Drawing for the job (mm, zero at the part's lowest x, y, z). A direction names the side the tool comes from. Round coordinates to 2 decimals unless told otherwise and drop trailing zeros. Order: outer loops, then holes, each group sorted by start corner. A loop starts at its lowest first (then second) coordinate and runs counter-clockwise, first axis right, second up. Notation, with made-up numbers: M 69.5,71.5 L 95.5,71.5 A25 cw 95.5,91.5 Z; hole C -33.75,84.5 d5. An arc over 180 degrees is marked long. One line per item, written item: value. Start each with the question number.
Item 1: Pin check, flat tips, straight feed: pin 1 (5.5 mm diameter, centred on x = 10, z = 3, fed in from +Y); pin 2 (2.5 mm diameter, centred on y = 1, z = 9.5, fed in from +X); pin 3 (5.5 mm diameter, centred on x = 11, z = 12.5, fed in from +Y); pin 4 (2.5 mm diameter, centred on x = 11, z = 11, fed in from -Y). Stop position of each tip, or through.
Item 2: Two-plate mould, pull along X, no slides. Class the marked faces 4, 5 and 6: +X half, -X half, draft (parallel to the pull), parting line (faces both ways), or undercut.
Item 3: Band-saw the part on D-D, the plane z = 8.25. Write the cut outline in (x, y).
Item 4: Probe L1, parallel to Y at x = 15.5, z = 6.5; L2, parallel to Y at x = 9.25, z = 6; L3, parallel to X at y = 1.5, z = 16.25. List the from-to ranges inside material, lowest first.
Item 5: Band-saw the part on B-B, the plane y = 2. Write the cut outline in (x, z).
Item 6: Tool access for the marked faces 1, 2 and 3: list every direction of +Z, -Z, +X, -X, +Y, -Y with a clear straight run to the whole face (end or side of a thin tool).
Item 7: Band-saw the part on C-C, the plane z = 11. Write the cut outline in (x, y), then the cut area to 3 significant figures.
Item 8: Band-saw the part on A-A, the plane x = 11. Write the cut outline in (y, z), then the cut area to 3 significant figures.
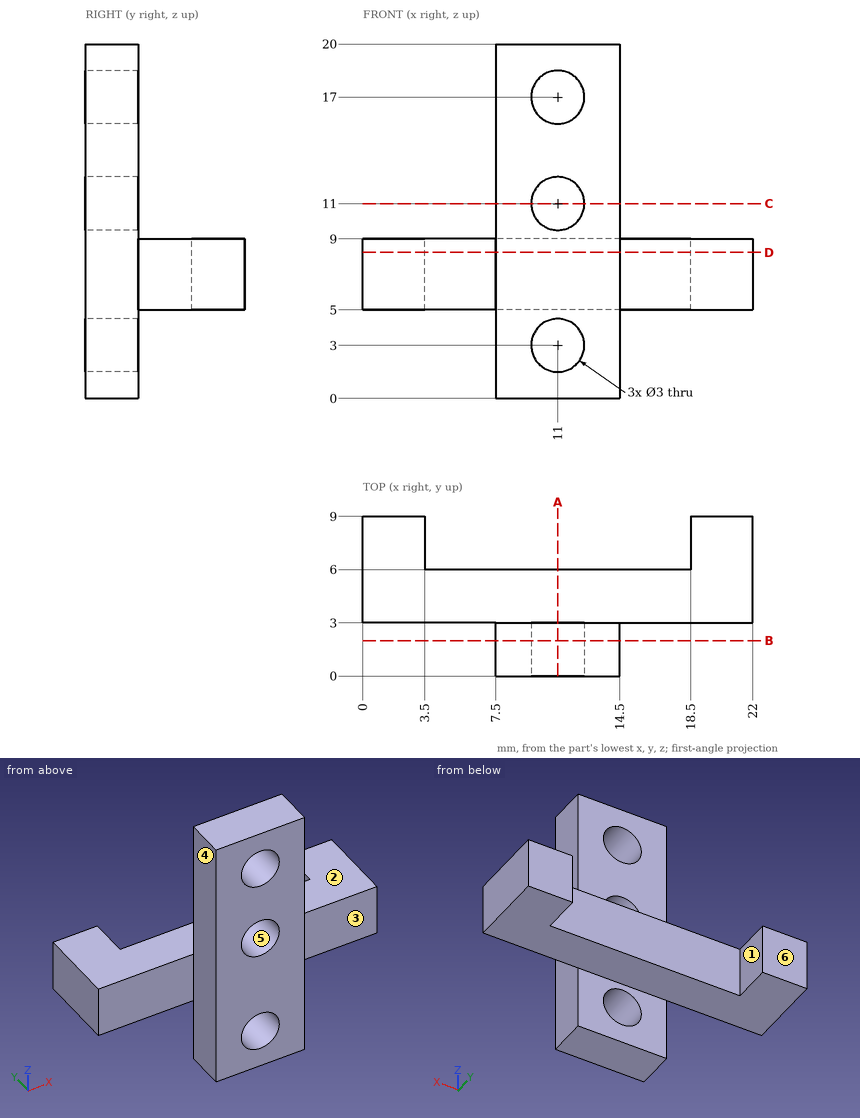
Output:
1. pin 1: stops at y = 6
1. pin 2: stops at x = 14.5
1. pin 3: stops at y = 3
1. pin 4: passes through
2. face 4: -X half
2. face 5: undercut
2. face 6: draft
3. outline: M 0,3 L 7.5,3 L 7.5,0 L 14.5,0 L 14.5,3 L 22,3 L 22,9 L 18.5,9 L 18.5,6 L 3.5,6 L 3.5,9 L 0,9 Z
4. L1: y = 3 to 6
4. L2: y = 0 to 6
4. L3: x = 7.5 to 9.7, 12.3 to 14.5
5. outline: M 7.5,0 L 14.5,0 L 14.5,20 L 7.5,20 Z; hole C 11,3 d3; hole C 11,11 d3; hole C 11,17 d3
6. face 1: +Z, -Z, +Y
6. face 2: +Z, +X, -X, +Y
6. face 3: +Z, -Z, +X, -Y
7. outline: M 7.5,0 L 9.5,0 L 9.5,3 L 7.5,3 Z; M 12.5,0 L 14.5,0 L 14.5,3 L 12.5,3 Z
7. area: 12.0 mm²
8. outline: M 0,0 L 3,0 L 3,1.5 L 0,1.5 Z; M 0,4.5 L 3,4.5 L 3,5 L 6,5 L 6,9 L 3,9 L 3,9.5 L 0,9.5 Z; M 0,12.5 L 3,12.5 L 3,15.5 L 0,15.5 Z; M 0,18.5 L 3,18.5 L 3,20 L 0,20 Z
8. area: 45.0 mm²
